Here's how the part is built. I have some questions about the finished solid (model axes, mm). Face numbers are marked on the shaded views. Give positions to 0.01 mm unless a question says otherwise; leave off trailing zeros. Write each loop counter-clockwise with the first axis right and the second up, starting at its lowest first coordinate (ties: lowest second). Pieces come first, ordered by that corner, then holes. Notation, with made-up numbers: (-15.75, -37.5) -> (36.25, -37.5) arc R30 ccw to (36.25, -9.5) -> close; hole circle Ø9 at (26, 89). An arc over 180 degrees is marked (long way). Use one line per item in the form item = value.
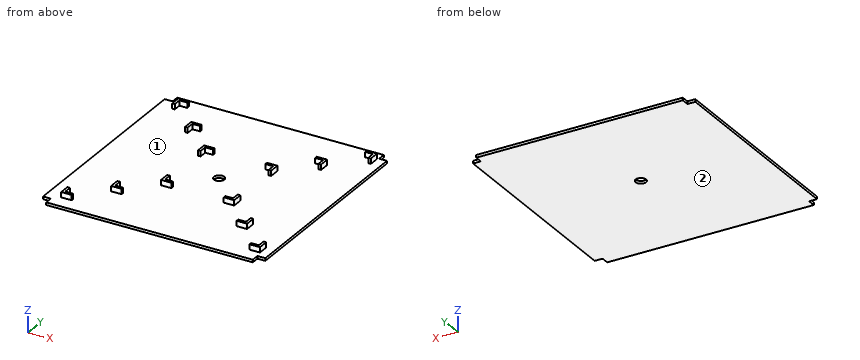
```python
from build123d import *

# Parameters (mm, degrees)
F0_R     = 25.4
F1_DEPTH = 12.7
F3_DEPTH = 25.4


with BuildPart() as f1:
    # F0 (on Top) → F1 (new body)
    with BuildSketch(Plane.XY):
        Polygon((-514.35, 488.95), (-552.45, 488.95), (-552.45, -514.35), (-514.35, -514.35), (-514.35, -552.45), (488.95, -552.45), (488.95, -514.35), (527.05, -514.35), (527.05, 488.95), (488.95, 488.95), (488.95, 527.05), (-514.35, 527.05), align=None)
        Circle(F0_R, mode=Mode.SUBTRACT)
    extrude(amount=F1_DEPTH)

    # F2 (on face) → F3 (join)
    with BuildSketch(Plane.XY.offset(12.7)):
        Polygon((-330.2, 330.2), (-330.2, 279.4), (-317.5, 279.4), (-317.5, 317.5), (-279.4, 317.5), (-279.4, 330.2), align=None)
        Polygon((-127, 177.8), (-177.8, 177.8), (-177.8, 127), (-165.1, 127), (-165.1, 165.1), (-127, 165.1), align=None)
        Polygon((-165.1, -127), (-177.8, -127), (-177.8, -177.8), (-127, -177.8), (-127, -165.1), (-165.1, -165.1), align=None)
        Polygon((177.8, 177.8), (127, 177.8), (127, 165.1), (165.1, 165.1), (165.1, 127), (177.8, 127), align=None)
        Polygon((330.2, 330.2), (279.4, 330.2), (279.4, 317.5), (317.5, 317.5), (317.5, 279.4), (330.2, 279.4), align=None)
        Polygon((177.8, -177.8), (177.8, -127), (165.1, -127), (165.1, -165.1), (127, -165.1), (127, -177.8), align=None)
        Polygon((482.6, 482.6), (431.8, 482.6), (431.8, 469.9), (469.9, 469.9), (469.9, 431.8), (482.6, 431.8), align=None)
        Polygon((-431.8, 482.6), (-482.6, 482.6), (-482.6, 431.8), (-469.9, 431.8), (-469.9, 469.9), (-431.8, 469.9), align=None)
        Polygon((-317.5, -279.4), (-330.2, -279.4), (-330.2, -330.2), (-279.4, -330.2), (-279.4, -317.5), (-317.5, -317.5), align=None)
        Polygon((-469.9, -431.8), (-482.6, -431.8), (-482.6, -482.6), (-431.8, -482.6), (-431.8, -469.9), (-469.9, -469.9), align=None)
        Polygon((330.2, -330.2), (330.2, -279.4), (317.5, -279.4), (317.5, -317.5), (279.4, -317.5), (279.4, -330.2), align=None)
        Polygon((431.8, -482.6), (482.6, -482.6), (482.6, -431.8), (469.9, -431.8), (469.9, -469.9), (431.8, -469.9), align=None)
    extrude(amount=F3_DEPTH)


solid = f1.part
```
Q1. If we mould it in two halves opening along Y, with no side actions, what happens to the marked faces 1 and 2? For each: +Y half, -Y half, draft (parallel to the pull), parting line (faces both ways), or undercut.
Result set:
face_1 = undercut
face_2 = draft
Q2. I want a section at D-D, the plane y = 301. Write out the boundary of the cut face in (x, z).
Result set:
outline = (-552.45, 0) -> (527.05, 0) -> (527.05, 12.7) -> (330.2, 12.7) -> (330.2, 38.1) -> (317.5, 38.1) -> (317.5, 12.7) -> (-317.5, 12.7) -> (-317.5, 38.1) -> (-330.2, 38.1) -> (-330.2, 12.7) -> (-552.45, 12.7) -> close
Q3. I want a section at A-A, the plane y = 0. Write out the boundary of the cut face in (x, z).
Result set:
outline = (-552.45, 0) -> (-25.4, 0) -> (-25.4, 12.7) -> (-552.45, 12.7) -> close; (25.4, 0) -> (527.05, 0) -> (527.05, 12.7) -> (25.4, 12.7) -> close
Q4. If I drill on line 1 along X through (y, z) = (-479.5, 14.5); line 2 along Y through (x, z) = (0, 3); line 3 along X through (y, z) = (139, 35), over which ranges is the centre line in solid material (lowest first)? Write a range as from..to.
Result set:
line_1 = -482.6..-431.8, 431.8..482.6
line_2 = -552.45..-25.4, 25.4..527.05
line_3 = -177.8..-165.1, 165.1..177.8
Q5. I want a section at C-C, the plane z = 24.5. Count the separate pieces of the cut face and the enclosed holes in it, and give its area (3 significant figures).
Result set:
separate_pieces = 12
enclosed_holes = 0
area = 13,500 mm2
Q6. Will these pins go through, and if not, where does the flat tip stop? pin 1 Ø2 at (y, z) = (403.5, 14.5) entering from -X; pin 2 Ø14 at (x, z) = (-542, 7) entering from +Y; pin 3 Ø20.5 at (x, z) = (294, 28.5) entering from -Y; pin 4 Ø7.5 at (x, z) = (137, 26) entering from +Y.
Result set:
pin_1 = through
pin_2 = 488.95
pin_3 = -330.2
pin_4 = 177.8
